Verification items for the finished model (mm, model axes). A direction names the side the tool comes from. Round coordinates to 2 decimals unless told otherwise and drop trailing zeros. Order: outer loops, then holes, each group sorted by start corner. A loop starts at its lowest first (then second) coordinate and runs counter-clockwise, first axis right, second up. Notation, with made-up numbers: (-13, 19) -> (17, 19) arc R12 cw to (17, 33) -> close; hole circle Ø1 at (53, -23.75). An arc over 180 degrees is marked (long way). Return JSON: item names as keys, results as strings. Group by question number.
1) Scan lines: L1, parallel to X at y = 6.5, z = 1.25; L2, parallel to Z at x = -3.5, y = 0; L3, parallel to Z at x = -1.25, y = 0. Record each from-to range of solid material in increasing order.
2) Depth check by flat-ended pin: pin 1 (6 mm diameter, centred on x = -3.5, y = 5, fed in from -Z); pin 2 (4 mm diameter, centred on x = -7.5, z = -0.5, fed in from +Y); pin 3 (1.5 mm diameter, centred on x = -7, z = -4, fed in from -Y). Enter the tip coordinate at first touch or a pass-through.
3) Tool access check on faces 5 (the flat face through (-11.75, -4, -3)), 6 (the cylindrical face through (-8.059, -2.681, 6.466)), 7 (the flat face through (-2.75, 6, -3)). Record the directions out of +Z, -Z, +X, -X, +Y, -Y that give a thin tool (end or side, any length) a straight path to the whole face; none if there is none.
4) Section check A-A on x = 0.25. Enter the section's corners in (y, z), plus the area to 3 significant figures.
5) Draft check along Y on faces 1 (the cylindrical face through (3.66, 1.847, 5.866)), 2 (the flat face through (0.038, -1.096, 6.914)), 3 (the flat face through (0.038, 5.44, 4.406)), 4 (the cylindrical face through (0.162, 2.285, 3.584)). Enter one of: pulls with the +Y half, pulls with the -Y half, needs draft (parallel to the pull), parting line crosses it, or undercut.
```python
from build123d import *

# Parameters (mm, degrees)
F2_SIZE2       = 0.75
F2_SIZE        = 0.75
F3_R           = 0.4
F7_DEPTH       = 2.75
F7_DEPTH_BACK  = 2.75
F8_R           = 0.4
F13_R          = 4.25
F14_DEPTH      = 25
F14_DEPTH_BACK = 44
F15_SIZE2      = 0.2
F15_SIZE       = 0.2


# Not quite as in the source:
# - an extrude ends at something that could not be found from the text; its depth is read off the source's solid


with BuildPart() as f1:
    # F0 (on Front) → F1 (revolve)
    with BuildSketch(Plane.XZ):
        Polygon((0, 6.15), (0, 0), (11.75, 0), (11.75, 7), (5.2, 7), (4.35, 6.15), (2.75, 6.15), align=None)
    revolve(axis=Axis((5.875, 0, 0), (-1, 0, 0)))

    # F2
    f2_edges = [f1.edges().sort_by_distance(p)[0] for p in [
        (11.75, 0, -7),
    ]]
    chamfer(f2_edges, length=F2_SIZE, length2=F2_SIZE2)

    # F3
    f3_edges = [f1.edges().sort_by_distance(p)[0] for p in [
        (4.35, 0, -6.15),
    ]]
    fillet(f3_edges, radius=F3_R)

    # F4: F1 across plane


with BuildPart() as f1_1:
    add(f1.part)
    add(f1.part.mirror(Plane.XZ))

    # F5: F1 across plane


with BuildPart() as f1_2:
    add(f1_1.part)
    add(f1_1.part.mirror(Plane.YZ))

    # F6 (on Right) → F7 (join, two sides)
    with BuildSketch(Plane.YZ) as f7_sk:
        Polygon((2.834367898, 7.5696559996), (-5.1383304446, 6.2394626031), (-7.9726983425, -1.3301933965), (-2.834367898, -7.5696559996), (5.1383304446, -6.2394626031), (7.9726983425, 1.3301933965), align=None)
    extrude(amount=F7_DEPTH)
    extrude(f7_sk.sketch, amount=-F7_DEPTH_BACK)

    # F8
    f8_edges = [f1_2.edges().sort_by_distance(p)[0] for p in [
        (-2.75, 0, -6.15),
        (2.75, 0, -6.15),
    ]]
    fillet(f8_edges, radius=F8_R)


with BuildPart() as f10:
    # F9 (on Top) → F10 (revolve)
    with BuildSketch(Plane.XY):
        Polygon((-5.5153914727, 9.7084684995), (-2.75, 6.9), (-1.9974731336, 9.7084684995), align=None)
    revolve(axis=Axis((-5.9099821374, 0, 0), (1, 0, 0)))


with BuildPart() as f11_1:
    # F11: instance of F10
    add(f10.part.mirror(Plane.YZ))


with BuildPart() as f1_3:
    add(f1_2.part)

    # F12: cut F10, F11_1
    add(f10.part, mode=Mode.SUBTRACT)
    add(f11_1.part, mode=Mode.SUBTRACT)

    # F13 (on face) → F14 (cut, two sides)
    with BuildSketch(Plane.YZ.offset(11.75)) as f14_sk:
        Circle(F13_R)
    extrude(amount=-F14_DEPTH, mode=Mode.SUBTRACT)
    extrude(f14_sk.sketch, amount=F14_DEPTH_BACK, mode=Mode.SUBTRACT)

    # F15
    f15_edges = [f1_3.edges().sort_by_distance(p)[0] for p in [
        (11.75, -4.25, 0),
        (-11.75, -4.25, 0),
    ]]
    chamfer(f15_edges, length=F15_SIZE, length2=F15_SIZE2)


solid = f1_3.part
```
Check result:
{
 "1": {"L1": "-11.38 to -4.82, -2.75 to 2.75, 4.82 to 11.38", "L2": "-6.15 to -4.25, 4.25 to 6.15", "L3": "-7.1 to -4.25, 4.25 to 7.1"},
 "2": {"pin 1": "z = -6.75", "pin 2": "y = 7", "pin 3": "y = -6.2"},
 "3": {"face 5": "+Z, -Z, -X, +Y, -Y", "face 6": "-X", "face 7": "none"},
 "4": {"outline": "(-7.97, -1.33) -> (-2.83, -7.57) -> (5.14, -6.24) -> (7.97, 1.33) -> (2.83, 7.57) -> (-5.14, 6.24) -> close; hole circle Ø8.5 at (0, 0)", "area": "113 mm^2"},
 "5": {"face 1": "parting line crosses it", "face 2": "pulls with the -Y half", "face 3": "pulls with the +Y half", "face 4": "undercut"}
}
